Geometry check sheet. Reference: drawing and pictorial views, mm from the part's lowest x, y, z. A direction names the side the tool comes from. Coordinates: 2 decimals unless noted, no trailing zeros. Loops run counter-clockwise (first coordinate to the right, second up) from the corner with the lowest first, then second, coordinate; pieces in that order, holes last. Notation, with made-up numbers: (43, 60) -> (70, 60) arc R11 ccw to (70, 74) -> close; hole circle Ø1 at (-38, 76.25). An arc over 180 degrees is marked (long way). Answer as a JSON object with one key per item and string values.
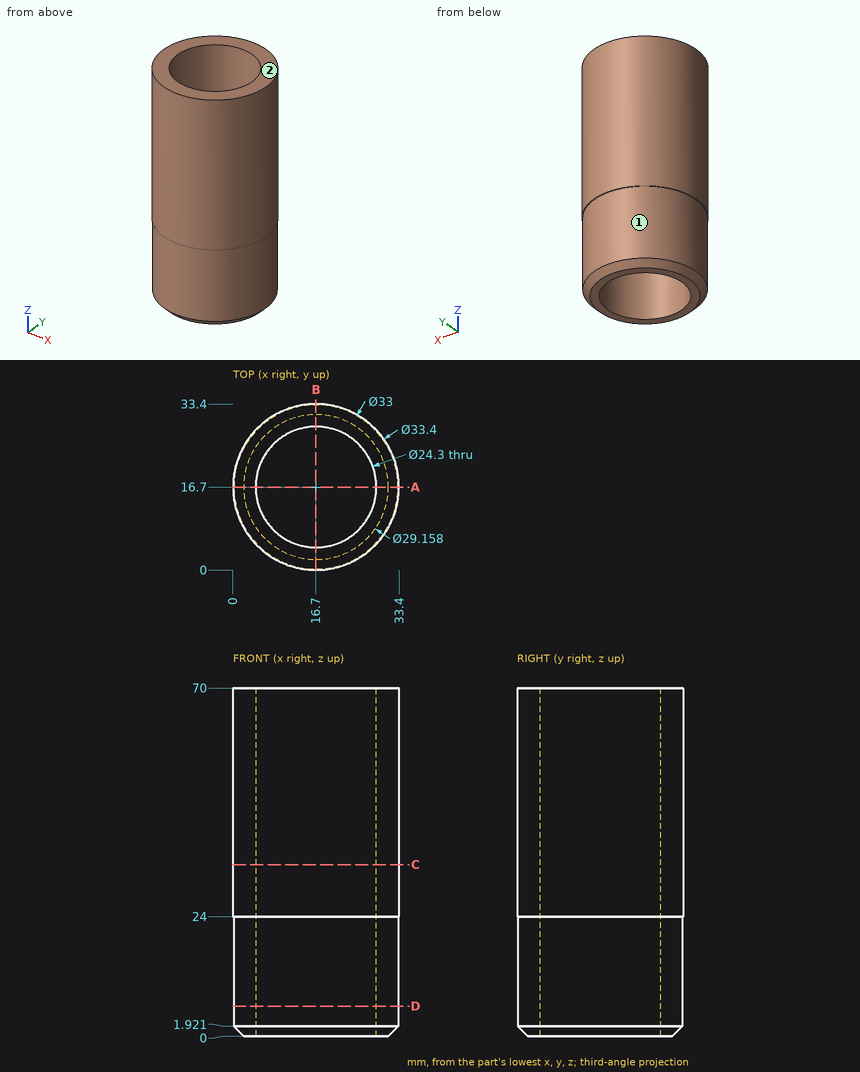
1. Thickness scan on probe 1 along Y at (x, z) = (16.7, 17); probe 2 along Y at (x, z) = (16.7, 34.5); probe 3 along X at (y, z) = (17.5, 32.5). Record the ranges inside material, lowest first. Write a range as from..to.
Evaluation:
{"probe 1": "y = 0.2..4.55, 28.85..33.2", "probe 2": "y = 0..4.55, 28.85..33.4", "probe 3": "x = 0.02..4.58, 28.82..33.38"}
2. Section check A-A, the plane y = 16.7. Record the boundary of the cut face in (x, z).
Evaluation:
{"outline": "(0, 24) -> (0.2, 24) -> (0.2, 1.92) -> (2.12, 0) -> (4.55, 0) -> (4.55, 70) -> (0, 70) -> close; (28.85, 0) -> (31.28, 0) -> (33.2, 1.92) -> (33.2, 24) -> (33.4, 24) -> (33.4, 70) -> (28.85, 70) -> close"}
3. Section check D-D, the plane z = 6. Record the boundary of the cut face in (x, y), then the cut area to 3 significant figures.
Evaluation:
{"outline": "circle Ø33 at (16.7, 16.7); hole circle Ø24.3 at (16.7, 16.7)", "area": "392 mm^2"}
4. Depth check by flat-ended pin: P1, Ø2, axis at y = 27.5, z = 61, coming from the +X side; P2, Ø5, axis at x = 30, z = 34, coming from the +Y side; P3, Ø6, axis at x = 8, z = 47, coming from the -Y side; P4, Ø6, axis at x = 8.5, y = 25, coming from the +Z side. Enter the tip coordinate at first touch or a pass-through.
Evaluation:
{"P1": "stops at x = 30.22", "P2": "stops at y = 29.44", "P3": "stops at y = 1", "P4": "stops at z = 70"}
5. Tool access check on the marked faces 1 and 2. Record the directions out of +Z, -Z, +X, -X, +Y, -Y that give a thin tool (end or side, any length) a straight path to the whole face; none if there is none.
Evaluation:
{"face 1": "-Z", "face 2": "+Z, +X, -X, +Y, -Y"}
6. Section check C-C, the plane z = 34.5. Record the boundary of the cut face in (x, y).
Evaluation:
{"outline": "circle Ø33.4 at (16.7, 16.7); hole circle Ø24.3 at (16.7, 16.7)"}
